The model under review builds one solid part; all positions refer to its coordinate system, in mm. A direction names the side the tool comes from. Coordinates: 2 decimals unless noted, no trailing zeros. Order: outer loops, then holes, each group sorted by start corner. A loop starts at its lowest first (then second) coordinate and runs counter-clockwise, first axis right, second up. Notation, with made-up numbers: (-2, -19.75) -> (18, -19.75) arc R37 cw to (18, 18.25) -> close; hole circle Ø9 at (48.5, 62.25). An arc over 180 degrees is marked (long way). Answer as CSV lines item,"result". Start each with the question number.
from build123d import *

# Parameters (mm, degrees)
F0_W     = 10
F0_H     = 4.0220445953
F0_W_2   = 90
F2_W     = 7.713583298
F2_H     = 4.518811591
F3_DEPTH = 10


with BuildPart() as f1:
    # F0 (on Top) → F1 (revolve)
    with BuildSketch(Plane.XY):
        with Locations((-17.5921608508, 6.033066893)):
            Rectangle(F0_W, F0_H)
        with Locations((-17.5921608508, 2.0110222977)):
            Rectangle(F0_W, F0_H)
        with Locations((32.4078391492, 2.0110222977)):
            Rectangle(F0_W_2, F0_H)
    revolve(axis=Axis((14.6210342646, 0, 0), (1, 0, 0)))

    # F2 (on Top) → F3 (cut)
    with BuildSketch(Plane.XY):
        with Locations((3.856791649, 0)):
            Rectangle(F2_W, F2_H)
    extrude(amount=F3_DEPTH, mode=Mode.SUBTRACT)


solid = f1.part
1) Consider section D-D (y = -7). Give the boundary of the cut face in (x, z), plus the area to 3 significant figures.
2) Consider section B-B (z = 1.5). Give the boundary of the cut face in (x, y), plus the area to 3 significant figures.
3) Insertion check: pin 1 Ø1.5 at (x, y) = (44.5, 1.5) entering from -Z; pin 2 Ø3.5 at (x, z) = (4.5, 1) entering from -Y; pin 3 Ø1 at (x, z) = (5.5, 2) entering from +Y. Each pin has a flat end and moves straight along its axis. Give the tip position at first contact, or say it passes through.
4) Mouldability with a two-part tool opening along X and no side actions: class faces 3 (the face through (-22.592, 0, 0)), 4 (the face through (-12.592, -2, 4)), 5 (the face through (7.714, 0, 2)), 6 (the face through (33.038, -0.872, -3.926)) as released by +X, released by -X, zero draft, split by the parting line, or undercut.
5) Consider section C-C (x = 51). Give the boundary of the cut face in (y, z).
6) Consider section A-A (y = 0). Give the boundary of the cut face in (x, z).
7) Tool access review of faces 1 (the face through (-17.522, -6.384, -4.895)), 2 (the face through (4, 2.259, 2)): name each direction out of +Z, -Z, +X, -X, +Y, -Y from which nothing blocks a thin tool from reaching the whole face with its end or side.
8) Wall thickness on L1, parallel to X at y = 0, z = 0.5; L2, parallel to X at y = -6.5, z = -1.75; L3, parallel to Y at x = 24.5, z = 0.25: over which ranges is each line inside the solid? List them lowest first. Write a range as [from, to].
Result:
1,outline,"(-22.59, -3.96) -> (-12.59, -3.96) -> (-12.59, 3.96) -> (-22.59, 3.96) -> close"
1,area,"79.3 mm2"
2,outline,"(-22.59, -7.9) -> (-12.59, -7.9) -> (-12.59, -3.73) -> (77.41, -3.73) -> (77.41, 3.73) -> (-12.59, 3.73) -> (-12.59, 7.9) -> (-22.59, 7.9) -> close; hole (0, -2.26) -> (7.71, -2.26) -> (7.71, 2.26) -> (0, 2.26) -> close"
2,area,"795 mm2"
3,pin 1,"z = -3.95"
3,pin 2,"y = -4.02"
3,pin 3,"y = 3.73"
4,face 3,"released by -X"
4,face 4,"released by +X"
4,face 5,"undercut"
4,face 6,"zero draft"
5,outline,"circle Ø8.04 at (0, 0)"
6,outline,"(-22.59, -8.04) -> (-12.59, -8.04) -> (-12.59, -4.02) -> (77.41, -4.02) -> (77.41, 4.02) -> (7.71, 4.02) -> (7.71, 0) -> (0, 0) -> (0, 4.02) -> (-12.59, 4.02) -> (-12.59, 8.04) -> (-22.59, 8.04) -> close"
7,face 1,"+X, -X"
7,face 2,"+Z"
8,L1,"[-22.59, 0], [7.71, 77.41]"
8,L2,"[-22.59, -12.59]"
8,L3,"[-4.01, 4.01]"
